Can you work these out from the model? Positions are in its coordinate system, mm. A direction names the side the tool comes from. Give positions to 0.01 mm unless a question says otherwise; leave off trailing zeros. Loops run counter-clockwise (first coordinate to the right, second up) from the corner with the lowest first, then second, coordinate; pieces in that order, holes last. Notation, with made-up numbers: (33, 64) - (75, 64) arc R19 ccw to (75, 80) - close; hole circle Ø11 at (69, 80). An arc over 180 degrees is marked (long way). Answer in a Markdown table with one row per item.
from build123d import *

# Parameters (mm, degrees)
EXTRUDE_1_DEPTH              = 3
HOLE_WIZARD_M3_1_D           = 2.5
HOLE_WIZARD_M3_1_CSINK_D     = 3.05
HOLE_WIZARD_M3_1_CSINK_ANGLE = 90


with BuildPart() as part:
    # 草图1 → 凸台-拉伸1 (new body)
    with BuildSketch(Plane(origin=(0, 0, 0), x_dir=(1, 0, 0), z_dir=(0, 1, 0))):
        with BuildLine():
            Line((4, -28), (4, 0))
            ThreePointArc((4, 0), (2.828427125, 2.828427125), (0, 4))
            Line((0, 4), (-12, 4))
            ThreePointArc((-12, 4), (-14.828427125, 2.828427125), (-16, 0))
            Line((-16, 0), (-16, -9.3))
            ThreePointArc((-16, -9.3), (-15.83835057, -10.425639773), (-15.366467551, -11.460300033))
            Line((-15.366467551, -11.460300033), (-3.366467551, -30.160300033))
            ThreePointArc((-3.366467551, -30.160300033), (1.125639773, -31.83835057), (4, -28))
        make_face()
        with BuildLine():
            Line((-8.683233775, -14.468627367), (-6.814876995, -17.380150016))
            ThreePointArc((-6.814876995, -17.380150016), (-6.09073132, -18.055035617), (-5.13164322, -18.3))
            Line((-5.13164322, -18.3), (0, -18.3))
            ThreePointArc((0, -18.3), (0.707106781, -18.007106781), (1, -17.3))
            Line((1, -17.3), (1, -4))
            ThreePointArc((1, -4), (0.707106781, -3.292893219), (0, -3))
            Line((0, -3), (-8, -3))
            ThreePointArc((-8, -3), (-8.707106781, -3.292893219), (-9, -4))
            Line((-9, -4), (-9, -13.388477351))
            ThreePointArc((-9, -13.388477351), (-8.919175285, -13.951297237), (-8.683233775, -14.468627367))
        make_face(mode=Mode.SUBTRACT)
    extrude(amount=EXTRUDE_1_DEPTH)

    # M3 螺纹孔1 (through all)
    with Locations(Plane(origin=(0, 3, 0), x_dir=(1, 0, 0), z_dir=(0, 1, 0))):
        with Locations((-12, 0), (-12, -9.3), (0, 0), (0, -21.3), (0, -28)):
            CounterSinkHole(HOLE_WIZARD_M3_1_D / 2, HOLE_WIZARD_M3_1_CSINK_D / 2, counter_sink_angle=HOLE_WIZARD_M3_1_CSINK_ANGLE)


solid = part.part
Q1. Imagine slicing it at A-A, the plane z = 5. Write out the boundary of the cut face in (x, y).
Checked values:
| item | result |
|---|---|
| outline | (-16, 0) - (-9, 0) - (-9, 3) - (-16, 3) - close; (1, 0) - (4, 0) - (4, 3) - (1, 3) - close |
Q2. Imagine slicing it at C-C, the plane z = 21.3. Write out the boundary of the cut face in (x, y) (3 decimals).
Checked values:
| item | result |
|---|---|
| outline | (-9.052, 0) - (-1.25, 0) - (-1.25, 2.725) - (-1.525, 3) - (-9.052, 3) - close; (1.25, 0) - (4, 0) - (4, 3) - (1.525, 3) - (1.25, 2.725) - close |
Q3. Imagine slicing it at B-B, the plane y = 1.85. Write out the boundary of the cut face in (x, z).
Checked values:
| item | result |
|---|---|
| outline | (-16, 0) arc R4 ccw to (-12, -4) - (0, -4) arc R4 ccw to (4, 0) - (4, 28) arc R4 ccw to (-3.37, 30.16) - (-15.37, 11.46) arc R4 ccw to (-16, 9.3) - close; hole circle Ø2.5 at (-12, 0); hole circle Ø2.5 at (-12, 9.3); hole (-9, 4) arc R1 ccw to (-8, 3) - (0, 3) arc R1 ccw to (1, 4) - (1, 17.3) arc R1 ccw to (0, 18.3) - (-5.13, 18.3) arc R2 ccw to (-6.81, 17.38) - (-8.68, 14.47) arc R2 ccw to (-9, 13.39) - close; hole circle Ø2.5 at (0, 0); hole circle Ø2.5 at (0, 21.3); hole circle Ø2.5 at (0, 28) |
Q4. Imagine slicing it at D-D, the plane z = 10. Count the separate pieces of the cut face and the enclosed holes in it, and give its area (3 significant figures).
Checked values:
| item | result |
|---|---|
| separate pieces | 3 |
| enclosed holes | 0 |
| area | 23.5 mm² |
Q5. For pin 1 (4 mm diameter, centred on x = -5, z = 18.5, fed in from -Y); pin 2 (1.5 mm diameter, centred on y = 0.5, z = 15.5, fed in from -X); pin 3 (0.9 mm diameter, centred on y = 1, z = 12.5, fed in from -X); pin 4 (1 mm diameter, centred on y = 2, z = 25, fed in from -X), each with a flat end and sliding along its axis, tell me the tip position at first contact or that it passes through.
Checked values:
| item | result |
|---|---|
| pin 1 | stops at y = 0 |
| pin 2 | stops at x = -13.26 |
| pin 3 | stops at x = -14.99 |
| pin 4 | stops at x = -7 |
Q6. On a 3-axis mill with a long thin cutter (end or side, diameter ignored), from which of +Z, -Z, +X, -X, +Y, -Y can I reach the whole of each face in a straight line? I mean faces 1 (the face through (1, 1, 11)), 2 (the face through (1.056, 1.479, 31.858)). Say none if no direction works.
Checked values:
| item | result |
|---|---|
| face 1 | +Y, -Y |
| face 2 | +Z, +Y, -Y |
Q7. If we mould it in two halves opening along X, with no side actions, what happens to faces 3 (the face through (-10.6, 0, 9.7)), 4 (the face through (-14.797, 1.479, -2.859)), 5 (the face through (-4, 1, 3))? For each: released by +X, released by -X, zero draft, split by the parting line, or undercut.
Checked values:
| item | result |
|---|---|
| face 3 | zero draft |
| face 4 | released by -X |
| face 5 | undercut |
Q8. If I drill on line 1 (Z direction, x = -12, y = 1.8); line 2 (X direction, y = 1.5, z = 21.3); line 3 (X direction, y = 2, z = 28), over which ranges is the centre line in solid material (lowest first)? Write a range as [from, to].
Checked values:
| item | result |
|---|---|
| line 1 | z = [-4, -1.25], [1.25, 8.05], [10.55, 16.71] |
| line 2 | x = [-9.05, -1.25], [1.25, 4] |
| line 3 | x = [-4.75, -1.25], [1.25, 4] |
